Check sheet for the drawn part. Datum: minimum x, y, z corner. Units: mm. Coordinates: 2 decimals unless noted, no trailing zeros. Write each loop counter-clockwise with the first axis right and the second up, starting at its lowest first coordinate (ties: lowest second). Pieces come first, ordered by that corner, then holes. Notation, with made-up numbers: (-34.5, 89) - (-25.5, 89) arc R13 cw to (-25.5, 98) - close; hole circle Ø10 at (18, 71). An arc over 180 degrees is marked (long way). Answer as CSV lines item,"result". Start each with the question number.
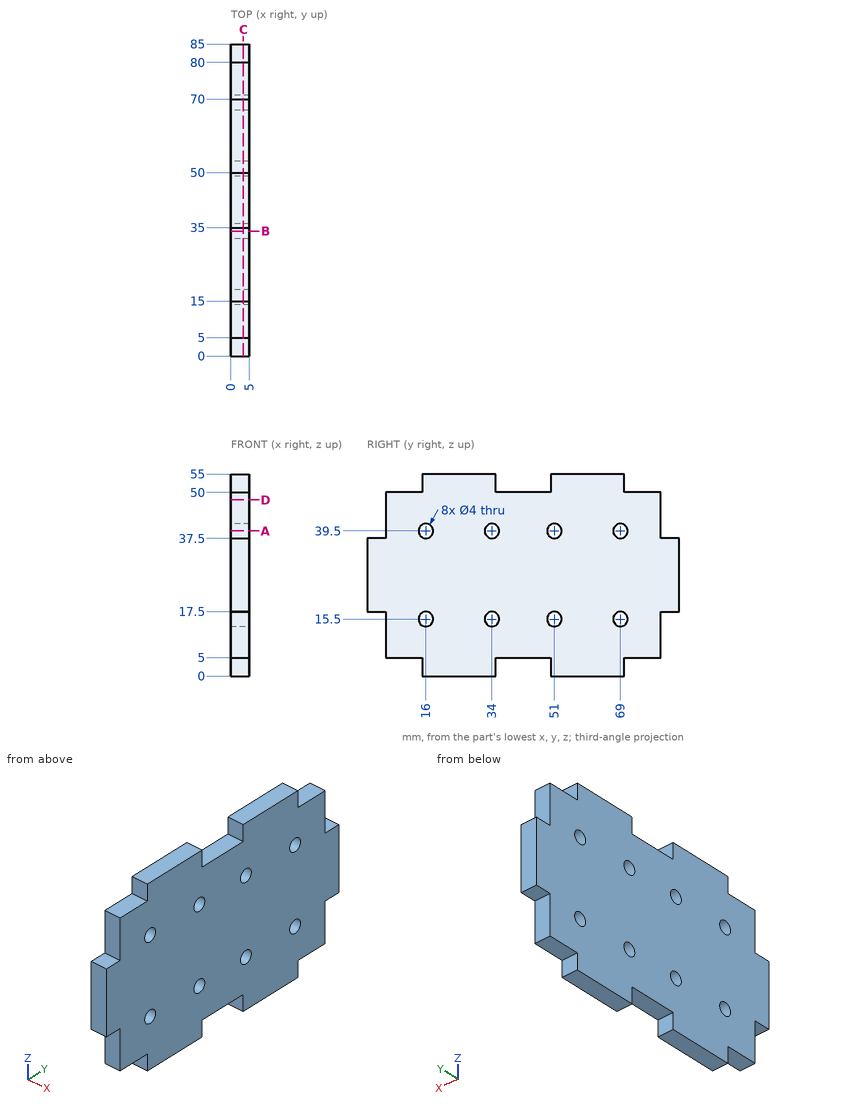
(1) Material ranges on probe 1 along Y at (x, z) = (1.15, 39.5); probe 2 along Z at (x, y) = (3.45, 69); probe 3 along Y at (x, z) = (3.5, 4.5), recorded low to high. Write a range as from..to.
(2) Cross-section at C-C on x = 3.45. State how many separate pieces and enclosed holes the cut face has, plus the area to 3 significant figures.
(3) Cross-section at A-A on z = 39.5. Record the boundary of the cut face in (x, y), plus the area to 3 significant figures.
(4) Cross-section at B-B on y = 34. Record the boundary of the cut face in (x, z), plus the area to 3 significant figures.
(5) Cross-section at D-D on z = 48. Record the boundary of the cut face in (x, y).
(6) Go/stop test with flat-tipped pins: P1, Ø2.5, axis at x = 3, z = 3.5, coming from the +Y side; P2, Ø2.5, axis at x = 2, z = 2.5, coming from the -Y side; P3, Ø1.5, axis at x = 3, y = 8.5, coming from the +Z side. Record where each tip stops, or that it passes through.
Checked values:
1,probe 1,"5..14, 18..32, 36..49, 53..67, 71..80"
1,probe 2,"0..13.5, 17.5..37.5, 41.5..55"
1,probe 3,"15..35, 50..70"
2,separate pieces,"1"
2,enclosed holes,"8"
2,area,"3,870 mm^2"
3,outline,"(0, 5) - (5, 5) - (5, 14) - (0, 14) - close; (0, 18) - (5, 18) - (5, 32) - (0, 32) - close; (0, 36) - (5, 36) - (5, 49) - (0, 49) - close; (0, 53) - (5, 53) - (5, 67) - (0, 67) - close; (0, 71) - (5, 71) - (5, 80) - (0, 80) - close"
3,area,"295 mm^2"
4,outline,"(0, 0) - (5, 0) - (5, 13.5) - (0, 13.5) - close; (0, 17.5) - (5, 17.5) - (5, 37.5) - (0, 37.5) - close; (0, 41.5) - (5, 41.5) - (5, 55) - (0, 55) - close"
4,area,"235 mm^2"
5,outline,"(0, 5) - (5, 5) - (5, 80) - (0, 80) - close"
6,P1,"y = 70"
6,P2,"y = 15"
6,P3,"z = 50"
